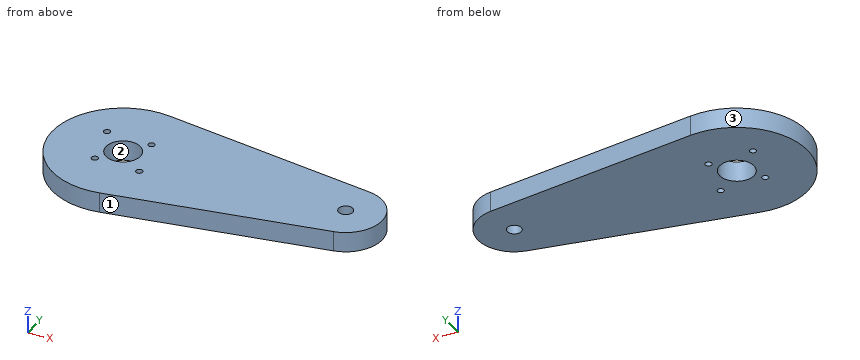
from build123d import *

# Parameters (mm, degrees)
SKETCH1_R           = 1.75
SKETCH1_R_2         = 4.25
SKETCH1_R_3         = 0.8
BOSS_EXTRUDE1_DEPTH = 5


with BuildPart() as part:
    # Sketch1 → Boss-Extrude1 (new body)
    with BuildSketch(Plane.XY):
        with BuildLine():
            Line((34.828288655, 68.520105857), (-18.109200177, 74.952234287))
            ThreePointArc((-18.109200177, 74.952234287), (-37.707923205, 56.929967705), (-16.825342518, 40.41240551))
            Line((-16.825342518, 40.41240551), (35.488558309, 50.756765343))
            ThreePointArc((35.488558309, 50.756765343), (42.736523537, 59.920116261), (34.828288655, 68.520105857))
        make_face()
        with Locations((33.74273446, 59.585813938)):
            Circle(SKETCH1_R, mode=Mode.SUBTRACT)
        with Locations((-20.22, 57.58)):
            Circle(SKETCH1_R_2, mode=Mode.SUBTRACT)
        with Locations((-27.101304543, 62.984641319)):
            Circle(SKETCH1_R_3, mode=Mode.SUBTRACT)
        with Locations((-16.050705268, 62.888434933)):
            Circle(SKETCH1_R_3, mode=Mode.SUBTRACT)
        with Locations((-13.338695457, 52.175358681)):
            Circle(SKETCH1_R_3, mode=Mode.SUBTRACT)
        with Locations((-24.389294732, 52.271565067)):
            Circle(SKETCH1_R_3, mode=Mode.SUBTRACT)
    extrude(amount=-BOSS_EXTRUDE1_DEPTH)


solid = part.part
Input: part model. Units: mm. Frame: model coordinates. Face numbers are marked on the shaded views. Coordinates: 2 decimals unless noted, no trailing zeros. Write each loop counter-clockwise with the first axis right and the second up, starting at its lowest first coordinate (ties: lowest second). Pieces come first, ordered by that corner, then holes. Notation, with made-up numbers: M 22.5,-29 L 35.5,-29 A26 ccw 35.5,7 Z; hole C 60,-14 d1. An arc over 180 degrees is marked long. Answer as a JSON object with one key per item and string values. Group by question number.
(1) Section B-B on z = -1.5. Output: boundary loops of the cut face in (x, y), plus the area to 3 significant figures.
(2) Section C-C on y = 66.5. Output: boundary loops of the cut face in (x, z).
(3) Contact query for flat-ended pins moving along their axis: P1, Ø1, axis at x = 5.5, z = -3.5, coming from the -Y side; P2, Ø2, axis at x = 11, z = -2.5, coming from the -Y side; P3, Ø1, axis at x = -10, z = -3.5, coming from the -Y side. Output: stop coordinate, or through.
(4) Section D-D on x = 28.5. Output: boundary loops of the cut face in (y, z).
(5) Mould query, pull axis Y, two halves, no side actions, for the marked faces 1, 2 and 3. Classes: pulls with the +Y half, pulls with the -Y half, needs draft (parallel to the pull), parting line crosses it, or undercut.
(6) Section A-A on x = -20.22. Output: boundary loops of the cut face in (y, z).
(7) Ray query, line 1 along X through (y, z) = (52.5, -1); line 2 along X through (y, z) = (59.5, -3.5); line 3 along X through (y, z) = (57, -0.3). Return the intervals inside material, ascending. Write a range as [from, to].
Result set:
{
 "1": {"outline": "M -18.11,74.95 A17.5 ccw long -16.83,40.41 L 35.49,50.76 A9 ccw 34.83,68.52 Z; hole C -27.1,62.98 d1.6; hole C -24.39,52.27 d1.6; hole C -20.22,57.58 d8.5; hole C -16.05,62.89 d1.6; hole C -13.34,52.18 d1.6; hole C 33.74,59.59 d3.5", "area": "1,980 mm2"},
 "2": {"outline": "M -35.28,-5 L 39.5,-5 L 39.5,0 L -35.28,0 Z"},
 "3": {"P1": "stops at y = 44.73", "P2": "stops at y = 45.72", "P3": "stops at y = 41.66"},
 "4": {"outline": "M 49.37,-5 L 69.29,-5 L 69.29,0 L 49.37,0 Z"},
 "5": {"face 1": "pulls with the -Y half", "face 2": "undercut", "face 3": "parting line crosses it"},
 "6": {"outline": "M 40.08,-5 L 53.33,-5 L 53.33,0 L 40.08,0 Z; M 61.83,-5 L 75.08,-5 L 75.08,0 L 61.83,0 Z"},
 "7": {"line 1": "x = [-36.97, -25.16], [-23.62, -14.07], [-12.61, 39.29]", "line 2": "x = [-37.61, -24.01], [-16.43, 31.99], [35.49, 42.74]", "line 3": "x = [-37.71, -24.43], [-16.01, 42.36]"}
}
